from build123d import *

# Parameters (mm, degrees)
ESQUISSE1_R        = 3.5
ESQUISSE1_R_2      = 2.25
BOSS_EXTRU_1_DEPTH = 27
CHANFREIN2_SIZE    = 0.5
CHANFREIN3_SIZE    = 0.5


with BuildPart() as part:
    # Esquisse1 → Boss.-Extru.1 (new body)
    with BuildSketch(Plane.XY):
        Circle(ESQUISSE1_R)
        Circle(ESQUISSE1_R_2, mode=Mode.SUBTRACT)
    extrude(amount=BOSS_EXTRU_1_DEPTH)

    # Chanfrein2
    chanfrein2_edges = [part.edges().sort_by_distance(p)[0] for p in [
        (-3.5, 0, 0),
        (-2.25, 0, 0),
    ]]
    chamfer(chanfrein2_edges, length=CHANFREIN2_SIZE)

    # Chanfrein3
    chanfrein3_edges = [part.edges().sort_by_distance(p)[0] for p in [
        (-3.5, 0, 27),
        (-2.25, 0, 27),
    ]]
    chamfer(chanfrein3_edges, length=CHANFREIN3_SIZE)


solid = part.part
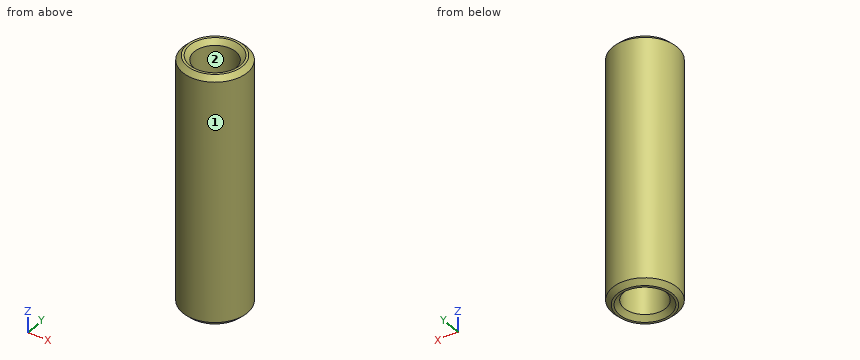
Input: part model. Units: mm. Frame: model coordinates. Face numbers are marked on the shaded views. Give positions to 0.01 mm unless a question says otherwise; leave off trailing zeros. Write each loop counter-clockwise with the first axis right and the second up, starting at its lowest first coordinate (ties: lowest second). Pieces come first, ordered by that corner, then holes. Notation, with made-up numbers: (-32.5, 32) -> (-6.5, 32) arc R33 ccw to (-6.5, 61) -> close; hole circle Ø4 at (79, 19.5). An arc over 180 degrees is marked (long way). Use one line per item in the form item = value. Start each with the question number.
1) Draft query along X for the marked faces 1 and 2. Return one class per face: pulls with the +X half, pulls with the -X half, needs draft (parallel to the pull), parting line crosses it, or undercut.
2) Section query C-C on z = 22.5. Return the cut outline in (x, y).
3) Section query A-A on x = 0. Return the cut outline in (y, z).
4) Ray query, probe 1 along Y at (x, z) = (0, 10.5); probe 2 along X at (y, z) = (1.25, 6); probe 3 along X at (y, z) = (-1.75, 17). Return the intervals inside material, ascending. Write a range as from..to.
5) Pin query (flat end, axial travel): pin 1 (1 mm diameter, centred on x = 1.5, z = 18.5, fed in from -Y); pin 2 (4 mm diameter, centred on y = -2.5, z = 17.5, fed in from +X); pin 3 (3 mm diameter, centred on y = -2.5, z = 3, fed in from -X). Return the tip coordinate at first contact, or that it passes through.
Outcome:
q1.face_1 = parting line crosses it
q1.face_2 = undercut
q2.outline = circle Ø7 at (0, 0); hole circle Ø4.5 at (0, 0)
q3.outline = (-3.5, 0.5) -> (-3, 0) -> (-2.75, 0) -> (-2.25, 0.5) -> (-2.25, 26.5) -> (-2.75, 27) -> (-3, 27) -> (-3.5, 26.5) -> close; (2.25, 0.5) -> (2.75, 0) -> (3, 0) -> (3.5, 0.5) -> (3.5, 26.5) -> (3, 27) -> (2.75, 27) -> (2.25, 26.5) -> close
q4.probe_1 = -3.5..-2.25, 2.25..3.5
q4.probe_2 = -3.27..-1.87, 1.87..3.27
q4.probe_3 = -3.03..-1.41, 1.41..3.03
q5.pin_1 = -3.35
q5.pin_2 = 3.46
q5.pin_3 = -3.35
